Answer from the drawing. Dimensions are ordinates in mm from the lowest x, y and z of the part. A direction names the side the tool comes from. Coordinates: 2 decimals unless noted, no trailing zeros. Loops run counter-clockwise (first coordinate to the right, second up) from the corner with the lowest first, then second, coordinate; pieces in that order, holes last. Notation, with made-up numbers: (56.25, 62) - (99.25, 62) arc R31 ccw to (99.25, 92) - close; hole circle Ø8 at (18, 20.25). An arc over 180 degrees is marked (long way). Use one line per item in the form item = value. Start each with the question number.
1) Each of these flat-tipped pins is pushed along its axis until it touches: P1, Ø1, axis at y = 6.5, z = 40, coming from the +X side; P2, Ø5, axis at x = 11.5, z = 30, coming from the +Y side; P3, Ø1.6, axis at y = 18, z = 49, coming from the -X side. Where does it stop, or does it pass through?
2) A cutting plane is placed at A-A (x = 9). Give the vertices of the cut face in (y, z).
3) A cutting plane is placed at D-D (y = 16.25). Give the vertices of the cut face in (x, z), and give its area (3 significant figures).
4) A cutting plane is placed at B-B (z = 2.7). Give the vertices of the cut face in (x, y), and give its area (3 significant figures).
5) The mould has two halves that part along X. Classify the marked faces 1, 2 and 3: released by +X, released by -X, zero draft, split by the parting line, or undercut.
6) A cutting plane is placed at C-C (y = 19). Give the vertices of the cut face in (x, z).
7) Which of the six approach directions +Z, -Z, +X, -X, +Y, -Y give full straight-line access (tool end or side, diameter ignored) to the marked faces 4 and 5?
8) Consider line 1 (X direction, y = 15, z = 10); line 2 (X direction, y = 14.5, z = 2.7); line 3 (Y direction, x = 23, z = 8). Determine where each line is inside the solid, lowest interval first.
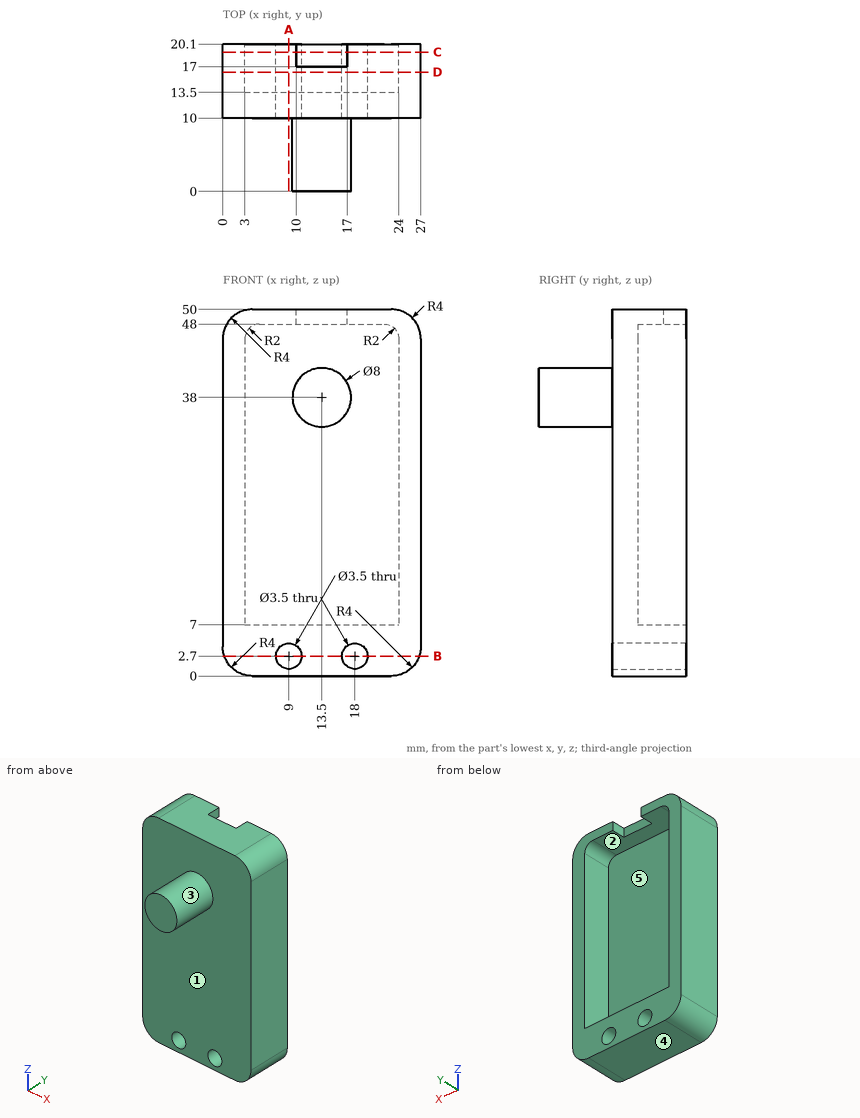
Found:
q1.P1 = 17.21
q1.P2 = 13.5
q1.P3 = 0.66
q2.outline = (10, 0) - (20.1, 0) - (20.1, 0.95) - (10, 0.95) - close; (10, 4.45) - (20.1, 4.45) - (20.1, 7) - (13.5, 7) - (13.5, 48) - (20.1, 48) - (20.1, 50) - (10, 50) - close
q3.outline = (0, 4) arc R4 ccw to (4, 0) - (23, 0) arc R4 ccw to (27, 4) - (27, 46) arc R4 ccw to (23, 50) - (4, 50) arc R4 ccw to (0, 46) - close; hole (3, 7) - (24, 7) - (24, 46) arc R2 ccw to (22, 48) - (5, 48) arc R2 ccw to (3, 46) - close; hole circle Ø3.5 at (9, 2.7); hole circle Ø3.5 at (18, 2.7)
q3.area = 458 mm^2
q4.outline = (0.22, 10) - (7.25, 10) - (7.25, 20.1) - (0.22, 20.1) - close; (10.75, 10) - (16.25, 10) - (16.25, 20.1) - (10.75, 20.1) - close; (19.75, 10) - (26.78, 10) - (26.78, 20.1) - (19.75, 20.1) - close
q4.area = 198 mm^2
q5.face_1 = zero draft
q5.face_2 = undercut
q5.face_3 = split by the parting line
q6.outline = (0, 4) arc R4 ccw to (4, 0) - (23, 0) arc R4 ccw to (27, 4) - (27, 46) arc R4 ccw to (23, 50) - (17, 50) - (17, 48) - (22, 48) arc R2 cw to (24, 46) - (24, 7) - (3, 7) - (3, 46) arc R2 cw to (5, 48) - (10, 48) - (10, 50) - (4, 50) arc R4 ccw to (0, 46) - close; hole circle Ø3.5 at (9, 2.7); hole circle Ø3.5 at (18, 2.7)
q7.face_4 = -Z, +X, -X, +Y, -Y
q7.face_5 = +Y
q8.line_1 = 0 to 3, 24 to 27
q8.line_2 = 0.22 to 7.25, 10.75 to 16.25, 19.75 to 26.78
q8.line_3 = 10 to 13.5
